Check sheet for the modelled part. Datum: model origin and axes. Units: mm. A direction names the side the tool comes from. Give positions to 0.01 mm unless a question says otherwise; leave off trailing zeros. Order: outer loops, then holes, each group sorted by start corner. A loop starts at its lowest first (then second) coordinate and runs counter-clockwise, first axis right, second up.
```python
from build123d import *

# Parameters (mm, degrees)
SKETCH2_R          = 1.25
CUT_EXTRUDE1_DEPTH = 5
SKETCH3_W          = 2.1
SKETCH3_H          = 11.085015624
CUT_EXTRUDE2_DEPTH = 5.5
CHAMFER1_SIZE      = 0.25


with BuildPart() as part:
    # Sketch1 → Revolve1 (revolve)
    with BuildSketch(Plane.XY, mode=Mode.PRIVATE) as revolve1_sk:
        Polygon((0, 0), (36, 0), (36, -2.5), (4, -2.5), (4, -1.75), (3.5, -1.75), (3.5, -2), (0, -2), align=None)
    revolve(revolve1_sk.sketch.rotate(Axis((0, 0, 0), (1, 0, 0)), 270), axis=Axis((0, 0, 0), (1, 0, 0)))

    # Sketch2 → Cut-Extrude1 (cut, symmetric)
    with BuildSketch(Plane.XY):
        with Locations((34, 0)):
            Circle(SKETCH2_R)
    extrude(amount=CUT_EXTRUDE1_DEPTH, both=True, mode=Mode.SUBTRACT)

    # Sketch3 → Cut-Extrude2 (cut)
    with BuildSketch(Plane(origin=(36, 0, 0), x_dir=(0, 0, -1), z_dir=(1, 0, 0))):
        Rectangle(SKETCH3_W, SKETCH3_H)
    extrude(amount=-CUT_EXTRUDE2_DEPTH, mode=Mode.SUBTRACT)

    # Chamfer1
    chamfer1_edges = [part.edges().sort_by_distance(p)[0] for p in [
        (0, 0, -2),
        (4, 0, -2.5),
        (3.5, 0, -1.75),
    ]]
    chamfer(chamfer1_edges, length=CHAMFER1_SIZE - 0.0001)  # a hair under: the kernel refuses the full size


solid = part.part
```
(1) Release check for a two-part mould opening along Z. For faces 1 (the face through (36, 0, 2)), 2 (the face through (33, -1, -1.05)), 3 (the face through (2, 2, 0)) record: released by +Z, released by -Z, zero draft, split by the parting line, or undercut.
Response values:
face 1: zero draft
face 2: undercut
face 3: split by the parting line
(2) Gauge pin test, flat ends, axial feed: pin 1 Ø1 at (x, y) = (22.5, -1.5) entering from +Z; pin 2 Ø2 at (x, y) = (6.5, 1.5) entering from -Z. Record the tip position at first contact, or that the pin passes through.
Response values:
pin 1: stops at z = 2.29
pin 2: stops at z = -2.45
(3) Set-up check for faces 4 (the face through (33, -1, 1.05)), 5 (the face through (4, 2, 0)), 6 (the face through (34.672, 1.054, -1.767)): record each of +Z, -Z, +X, -X, +Y, -Y from which the full face is reachable in a straight line by a thin tool's end or side.
Response values:
face 4: +X, +Y, -Y
face 5: none
face 6: +Z, -Z
(4) Cross-section at B-B on x = 34. Enter the section's corners in (y, z).
Response values:
outline: (-2.27, -1.05) arc R2.5 ccw to (-1.25, -2.17) - (-1.25, -1.05) - close; (-2.27, 1.05) - (-1.25, 1.05) - (-1.25, 2.17) arc R2.5 ccw to start; (1.25, -2.17) arc R2.5 ccw to (2.27, -1.05) - (1.25, -1.05) - close; (1.25, 1.05) - (2.27, 1.05) arc R2.5 ccw to (1.25, 2.17) - close
(5) Cross-section at D-D on x = 25.5. Enter the section's corners in (y, z), then the cut area to 3 significant figures.
Response values:
outline: circle Ø5 at (0, 0)
area: 19.6 mm2
(6) Material ranges on L1, parallel to X at y = 1.1, z = -0.6; L2, parallel to X at y = -0.85, z = -2.3; L3, parallel to Y at x = 23, z = -1.1 (3 decimals), recorded low to high.
Response values:
L1: x = 0 to 30.5
L2: x = 4.2 to 33.08, 34.92 to 36
L3: y = -2.245 to 2.245
(7) Cross-section at A-A on y = 0. Count the separate pieces of the cut face and the enclosed holes in it, then the cut area to 3 significant figures.
Response values:
separate pieces: 3
enclosed holes: 0
area: 157 mm2
